Design review of the part built by this model. Coordinates are the model's own, in mm. Face numbers are marked on the shaded views. Round coordinates to 2 decimals unless told otherwise and drop trailing zeros. Loops run counter-clockwise (first coordinate to the right, second up) from the corner with the lowest first, then second, coordinate; pieces in that order, holes last. Notation, with made-up numbers: (-10, -39) -> (0, -39) arc R11 cw to (0, -19) -> close; hole circle Ø4 at (24, 55). An arc over 180 degrees is marked (long way). Answer as CSV lines item,"result". Start each with the question number.
(1) Take a section at C-C, the plane x = -1.5. Write out the cut boundary in (y, z).
(2) To check wall thickness, follow line 1 (Z direction, x = -0.7, y = -0.5); line 2 (Y direction, x = -3.9, z = -14); line 3 (Y direction, x = -1.2, z = -12). State the ranges of each line that lie inside material, in increasing order. Write a range as from..to.
(3) Take a section at D-D, the plane y = -15. Write out the cut boundary in (x, z), and give its area (3 significant figures).
(4) Draft analysis for pull direction Z (two halves, no side actions). For the marked faces 1, 2 and 3, state which applies: +Z half, -Z half, draft (parallel to the pull), parting line (faces both ways), or undercut.
(5) Take a section at A-A, the plane y = 0. Write out the cut boundary in (x, z).
(6) For P1, Ø0.8, axis at x = -0.5, z = -1, coming from the -Y side; P2, Ø1.1, axis at x = -0.5, z = 1, coming from the +Y side; P3, Ø0.5, axis at x = -0.5, y = -3, coming from the -Z side, all flat-tipped, find the tip position at first contact; note any pin that passes through.
(7) Take a section at B-B, the plane z = 0. Write out the cut boundary in (x, y).
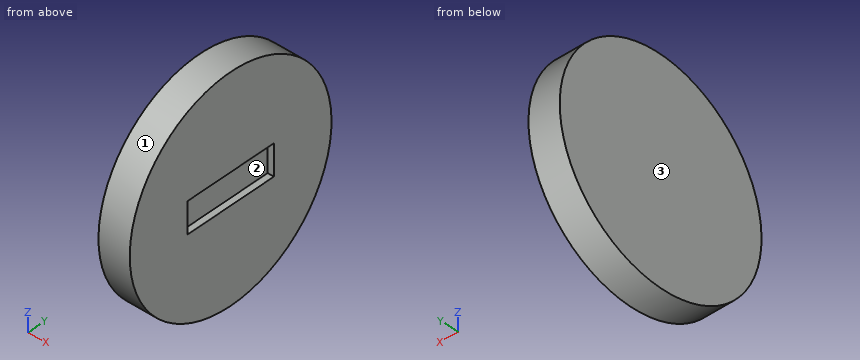
from build123d import *

# Parameters (mm, degrees)
SKETCH1_R           = 17.5
SKETCH1_W           = 5
SKETCH1_H           = 15
BOSS_EXTRUDE1_DEPTH = 5
SKETCH1_3_W         = 5
SKETCH1_3_H         = 15
CUT_EXTRUDE1_DEPTH  = 1


with BuildPart() as part:
    # Sketch1 → Boss-Extrude1 (new body)
    # profile 1 of 2: a face of its own
    with BuildSketch(Plane(origin=(0, 0, 0), x_dir=(0, 0, -1), z_dir=(1, 0, 0))):
        Circle(SKETCH1_R)
        Rectangle(SKETCH1_W, SKETCH1_H, mode=Mode.SUBTRACT)
    # profile 2 of 2: a face of its own
    with BuildSketch(Plane(origin=(0, 0, 0), x_dir=(0, 0, -1), z_dir=(1, 0, 0))):
        Rectangle(SKETCH1_W, SKETCH1_H)
    extrude(amount=-BOSS_EXTRUDE1_DEPTH)

    # Sketch1_3 → Cut-Extrude1 (cut)
    with BuildSketch(Plane(origin=(0, 0, 0), x_dir=(0, 0, -1), z_dir=(1, 0, 0))):
        Rectangle(SKETCH1_3_W, SKETCH1_3_H)
    extrude(amount=-CUT_EXTRUDE1_DEPTH, mode=Mode.SUBTRACT)


solid = part.part
The answers:
1,outline,"circle Ø35 at (0, 0)"
2,line 1,"-17.49..-2.5, 2.5..17.49"
2,line 2,"-10.5..10.5"
2,line 3,"-12.74..12.74"
3,outline,"(-5, -9.01) -> (0, -9.01) -> (0, 9.01) -> (-5, 9.01) -> close"
3,area,"90.1 mm²"
4,face 1,"parting line"
4,face 2,"undercut"
4,face 3,"draft"
5,outline,"(-5, -17.5) -> (0, -17.5) -> (0, -2.5) -> (-1, -2.5) -> (-1, 2.5) -> (0, 2.5) -> (0, 17.5) -> (-5, 17.5) -> close"
6,P1,"y = -17.49"
6,P2,"y = 17.49"
6,P3,"z = -17.28"
7,outline,"(-5, -17.5) -> (0, -17.5) -> (0, -7.5) -> (-1, -7.5) -> (-1, 7.5) -> (0, 7.5) -> (0, 17.5) -> (-5, 17.5) -> close"
